Design review of the part shown in the three views and the two pictorial views. Dimensions are in mm from the part's minimum x, y and z. A direction names the side the tool comes from. Coordinates: 2 decimals unless noted, no trailing zeros. Write each loop counter-clockwise with the first axis right and the second up, starting at its lowest first coordinate (ties: lowest second). Pieces come first, ordered by that corner, then holes. Notation, with made-up numbers: M -37,63.25 L -32,63.25 A26 ccw -32,101.25 Z; hole C 26,53 d9. An arc over 180 degrees is marked long. Answer as a JSON object with one key per item and string values.
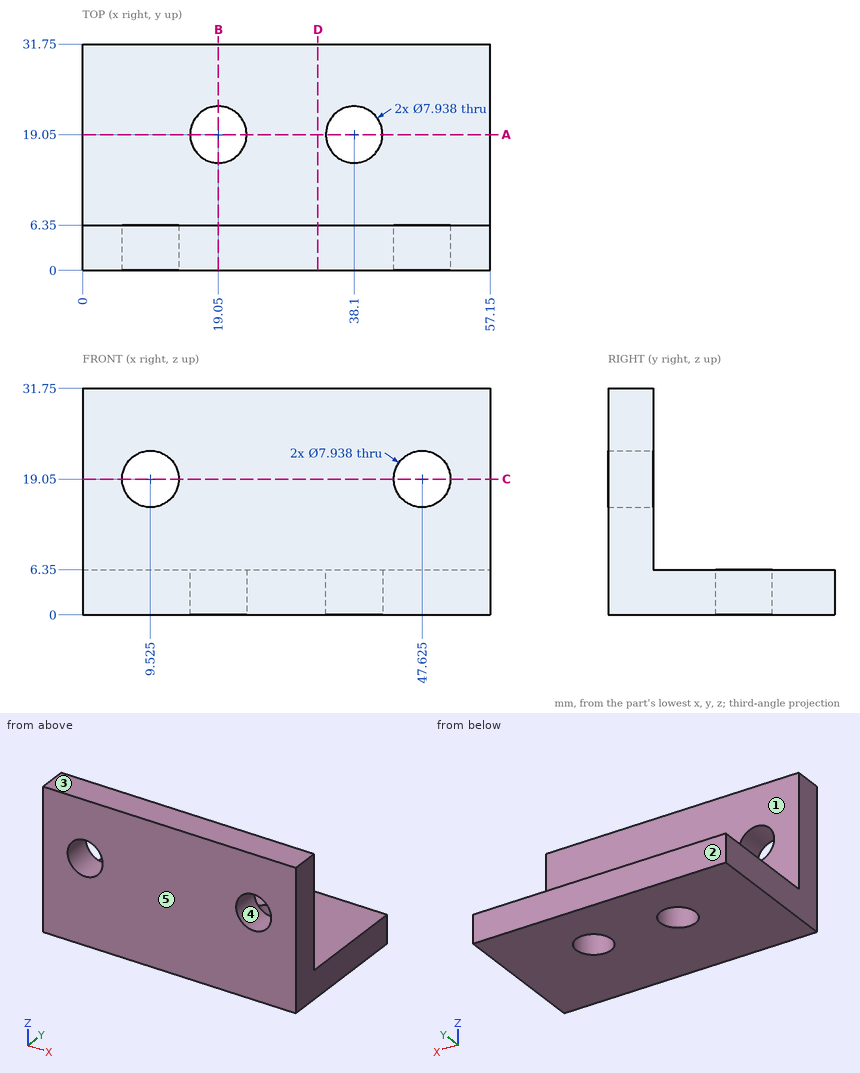
(1) Add section B-B on x = 19.05. Give the boundary of the cut face in (y, z).
Results list:
{"outline": "M 0,0 L 15.08,0 L 15.08,6.35 L 6.35,6.35 L 6.35,31.75 L 0,31.75 Z; M 23.02,0 L 31.75,0 L 31.75,6.35 L 23.02,6.35 Z"}
(2) Add section A-A on y = 19.05. Give the boundary of the cut face in (x, z), and give its area (3 significant figures).
Results list:
{"outline": "M 0,0 L 15.08,0 L 15.08,6.35 L 0,6.35 Z; M 23.02,0 L 34.13,0 L 34.13,6.35 L 23.02,6.35 Z; M 42.07,0 L 57.15,0 L 57.15,6.35 L 42.07,6.35 Z", "area": "262 mm²"}
(3) Add section C-C on z = 19.05. Give the boundary of the cut face in (x, y).
Results list:
{"outline": "M 0,0 L 5.56,0 L 5.56,6.35 L 0,6.35 Z; M 13.49,0 L 43.66,0 L 43.66,6.35 L 13.49,6.35 Z; M 51.59,0 L 57.15,0 L 57.15,6.35 L 51.59,6.35 Z"}
(4) Add section D-D on x = 33. Give the boundary of the cut face in (y, z).
Results list:
{"outline": "M 0,0 L 31.75,0 L 31.75,6.35 L 6.35,6.35 L 6.35,31.75 L 0,31.75 Z"}
(5) Wall thickness on line 1 along X through (y, z) = (19, 1); line 2 along X through (y, z) = (5.25, 19.05); line 3 along Z through (x, y) = (27.5, 30.5): over which ranges is each line inside the solid? List them lowest first. Write a range as from..to.
Results list:
{"line 1": "0..15.08, 23.02..34.13, 42.07..57.15", "line 2": "0..5.56, 13.49..43.66, 51.59..57.15", "line 3": "0..6.35"}
(6) For pin 1 Ø10.5 at (x, y) = (19.05, 19.05) entering from -Z; pin 2 Ø1.5 at (x, y) = (51, 25) entering from +Z; pin 3 Ø8 at (x, z) = (28, 16) entering from +Y, all flat-tipped, find the tip position at first contact; note any pin that passes through.
Results list:
{"pin 1": "z = 0", "pin 2": "z = 6.35", "pin 3": "y = 6.35"}
(7) Draft analysis for pull direction Z (two halves, no side actions). For the marked faces 3, 4 and 5, state which applies: released by +Z, released by -Z, zero draft, split by the parting line, or undercut.
Results list:
{"face 3": "released by +Z", "face 4": "undercut", "face 5": "zero draft"}
(8) For the marked faces 1 and 2, list the 3-axis set-ups (+Z, -Z, +X, -X, +Y, -Y) from which the entire face can be reached by the end or side of a thin tool; tool diameter is ignored.
Results list:
{"face 1": "+Z, +X, -X, +Y", "face 2": "+Z, -Z, +X, -X, +Y"}
